Check sheet for the drawn part. Datum: minimum x, y, z corner. Units: mm. Coordinates: 2 decimals unless noted, no trailing zeros. Order: outer loops, then holes, each group sorted by start corner. A loop starts at its lowest first (then second) coordinate and runs counter-clockwise, first axis right, second up. Notation, with made-up numbers: (79.5, 19) - (106.5, 19) arc R19 ccw to (106.5, 33) - close; hole circle Ø10 at (16.25, 73). An arc over 180 degrees is marked (long way). Answer as CSV lines item,"result". Start each with the question number.
1. Section check A-A (z = 12.7). Record the cut outline in (x, y).
2. Section check D-D (y = 6.5). Record the cut outline in (x, z), and give its area (3 significant figures).
3. Section check C-C (x = 9). Record the cut outline in (y, z).
4. Material ranges on L1, parallel to Z at x = 28.5, y = 2.5; L2, parallel to X at y = 2.25, z = 12.7; L3, parallel to Y at x = 17, z = 2, recorded low to high. Write a range as [from, to].
5. Section check B-B (y = 1.25). Record the cut outline in (x, z).
6. Go/stop test with a flat-tipped pin: pin 1 (1.5 mm diameter, centred on x = 24.5, z = 4, fed in from +Y). Record where the tip stops, or that it passes through.
7. Mould release check, pull along X, two halves, no side actions. Record for the marked faces 1, 2 and 3: pulls with the +X half, pulls with the -X half, needs draft (parallel to the pull), parting line crosses it, or undercut.
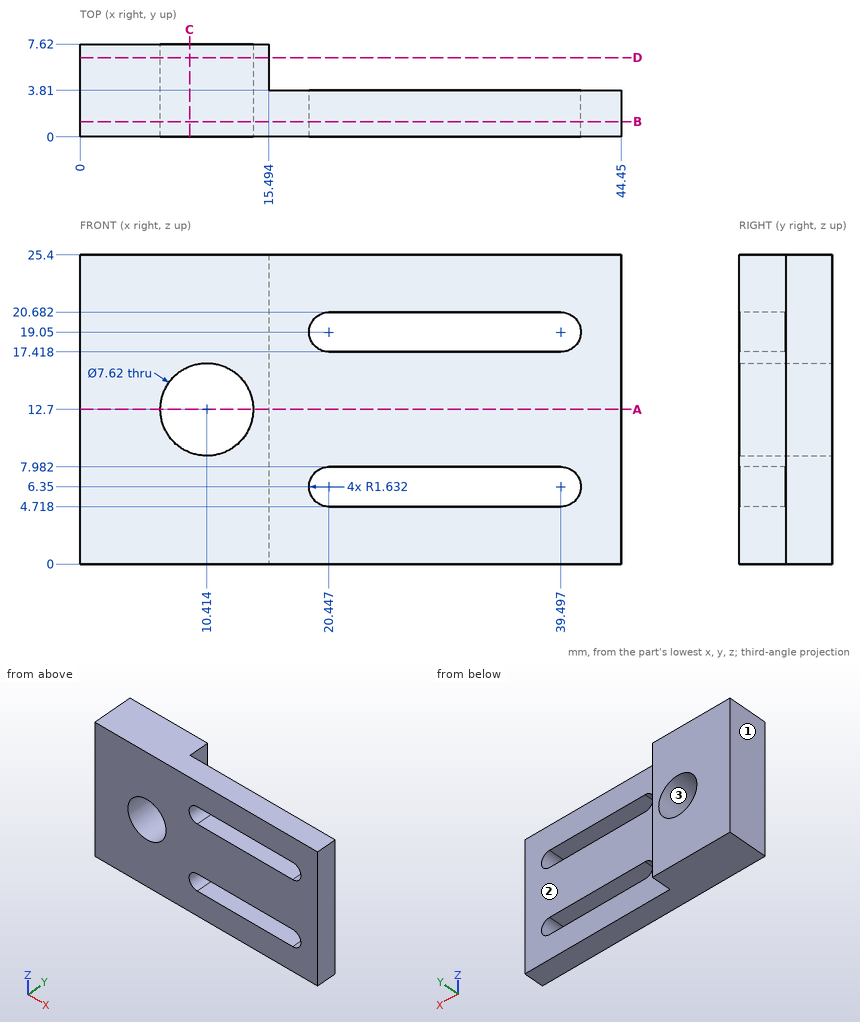
Evaluation:
1,outline,"(0, 0) - (6.6, 0) - (6.6, 7.62) - (0, 7.62) - close; (14.22, 0) - (44.45, 0) - (44.45, 3.81) - (15.49, 3.81) - (15.49, 7.62) - (14.22, 7.62) - close"
2,outline,"(0, 0) - (15.49, 0) - (15.49, 25.4) - (0, 25.4) - close; hole circle Ø7.62 at (10.41, 12.7)"
2,area,"348 mm²"
3,outline,"(0, 0) - (7.62, 0) - (7.62, 9.16) - (0, 9.16) - close; (0, 16.24) - (7.62, 16.24) - (7.62, 25.4) - (0, 25.4) - close"
4,L1,"z = [0, 4.72], [7.98, 17.42], [20.68, 25.4]"
4,L2,"x = [0, 6.6], [14.22, 44.45]"
4,L3,"y = [0, 3.81]"
5,outline,"(0, 0) - (44.45, 0) - (44.45, 25.4) - (0, 25.4) - close; hole circle Ø7.62 at (10.41, 12.7); hole (20.45, 4.72) - (39.5, 4.72) arc R1.63 ccw to (39.5, 7.98) - (20.45, 7.98) arc R1.63 ccw to start; hole (20.45, 17.42) - (39.5, 17.42) arc R1.63 ccw to (39.5, 20.68) - (20.45, 20.68) arc R1.63 ccw to start"
6,pin 1,"stops at y = 3.81"
7,face 1,"pulls with the -X half"
7,face 2,"needs draft"
7,face 3,"undercut"
